Work out the finished part from the listing and answer in its coordinate system (mm). Face numbers are marked on the shaded views. A direction names the side the tool comes from. Give positions to 0.01 mm unless a question says otherwise; leave off trailing zeros. Write each loop counter-clockwise with the first axis right and the second up, starting at its lowest first coordinate (ties: lowest second). Pieces come first, ordered by that corner, then holes.
1) A tool of negligible diameter and unlimited length cuts with its end or side. For the marked faces 1, 2 and 3, from which of +Z, -Z, +X, -X, +Y, -Y can it reach the whole face along a straight path? Write none if from no direction.
2) Given pin 1 Ø8 at (y, z) = (19, 56) entering from +X; pin 2 Ø6 at (x, z) = (20, 60) entering from -Y; pin 3 Ø2 at (x, z) = (37.5, 40) entering from -Y, each flat-ended and moving along its own axis, determine where each tip first touches the part or whether it passes through.
3) Find section C-C (z = 43.5). Determine the outline of the cut face in (x, y).
4) Find section D-D (y = 76). Determine the outline of the cut face in (x, z), plus the area to 3 significant figures.
5) Find section A-A (z = 25). Determine the outline of the cut face in (x, y).
6) Find section B-B (y = 8). Determine the outline of the cut face in (x, z).
7) Straight lines are drawn through the part: probe 1 along Z at (x, y) = (-5.5, 17); probe 2 along Z at (x, y) = (-4, 13); probe 3 along X at (y, z) = (67, 14.5). For each, find the intervals that lie inside material, in ascending order.
Autodesk Inventor part; units mm, degrees
ref_plane "Work Plane1" through (0, 0, 62.5) normal (0, 0, -1) x (-1, 0, 0)
ref_plane "Work Plane2" through (-10, 0, 62.5) normal (-0.9866, 0.1632, 0) x (-0.1632, -0.9866, 0)
ref_plane "YZ Plane" through (0, 0, 0) normal (1, 0, 0) x (0, 1, 0)
sketch "Sketch1" plane through (0, 0, 0) normal (0, 0, 1) x (1, 0, 0)
  arc A0 (45, 98) -> (0, 0) centre (139.9137, -4.9145) ccw
  line L0 (45, 98) -> (45, 93)
  line L1 (0, 0) -> (5, 0)
  arc A1 (45, 93) -> (5, 0) centre (144.908, -5.0734) ccw
  dimension "d0" = 140
  dimension "d1" = 98
  dimension "d3" = 45
  dimension "d4" = 5
  dimension "d5" = 5
  dimension "d6" = 140
extrude "Extrusion1" add sketch "Sketch1" along normal blind 125
ref_plane "Work Plane1" through (0, 0, 62.5) normal (0, 0, -1) x (-1, 0, 0)
sketch "Sketch3" plane through (0, 0, 62.5) normal (0, 0, -1) x (-1, 0, 0)
  arc A0 (0, 0) -> (-45, 98) centre (-139.9137, -4.9145) ccw
  line L0 (0, 0) -> (10, 0)
  arc A1 (10, 0) -> (-45, 98) centre (-152.788, -26.9269) ccw
  arc A2 (0, 0) -> (-45, 98) centre (-139.9137, -4.9145) ccw
  dimension "d19" = 10
  dimension "d20" = 165
extrude "Extrusion3" add sketch "Sketch3" along normal mid plane 85
ref_plane "Work Plane2" through (-10, 0, 62.5) normal (-0.9866, 0.1632, 0) x (-0.1632, -0.9866, 0)
sketch "Sketch2" plane through (-10, 0, 62.5) normal (-0.9866, 0.1632, 0) x (-0.1632, -0.9866, 0)
  circle A0 centre (-20.6619, -35) radius 4
  circle A1 centre (-72.6619, -35) radius 4
  circle A2 centre (-20.6619, 35) radius 4
  circle A3 centre (-72.6619, 35) radius 4
  line L0 (0, 42.5) -> (0, -42.5)
  line L1 (-72.6619, 35) -> (-20.6619, 35) construction
  line L2 (-20.6619, 35) -> (-20.6619, -35) construction
  line L3 (-20.6619, -35) -> (-72.6619, -35) construction
  line L4 (-72.6619, -35) -> (-72.6619, 35) construction
  line L5 (-105.6619, -42.5) -> (-105.6619, 42.5)
  point P0 (0, 0)
  point P1 (-20.6619, 0)
  point P2 (0, 0)
  dimension "d9" = 8
  dimension "d10" = 8
  dimension "d12" = 52
  dimension "d14" = 8
  dimension "d15" = 8
  dimension "d16" = 70
  dimension "d23" = 33
extrude "Extrusion2" cut sketch "Sketch2" against normal through all
sketch "Sketch4" plane through (-10, 0, 62.5) normal (-0.9866, 0.1632, 0) x (-0.1632, -0.9866, 0)
  circle A0 centre (-38, 0) radius 5
  line L0 (0, 42.5) -> (0, -42.5)
  point P0 (-1.6319, -62.5)
  point P1 (0, 0)
  dimension "d24" = 10
  dimension "d25" = 38
extrude "Extrusion4" cut sketch "Sketch4" against normal through all
properties part number "SJ009" material "ABS Plastic"
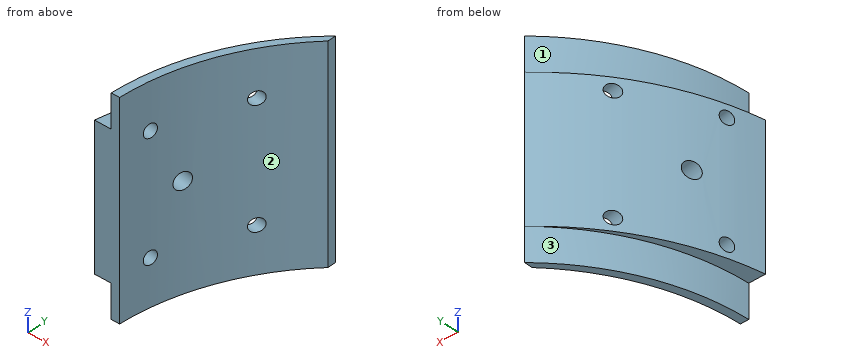
Results:
1. face 1: +Z, -X, +Y
1. face 2: +Z, -Z, +X, -Y
1. face 3: -Z, -X, +Y
2. pin 1: stops at x = 7.75
2. pin 2: stops at y = 51.84
2. pin 3: stops at y = 83.51
3. outline: (-10, 0) - (5, 0) arc R140 cw to (45, 93) - (45, 98) arc R165 ccw to start
4. outline: (23.83, 20) - (25.66, 20) - (25.66, 0) - (30.77, 0) - (30.77, 125) - (25.66, 125) - (25.66, 105) - (23.83, 105) - close
4. area: 795 mm2
5. outline: (-10, 0) - (5, 0) arc R140 cw to (6.36, 15.07) - (-6.22, 17.15) arc R165 ccw to start; (-4.42, 23.18) - (7.4, 21.23) arc R140 cw to (23.66, 64.92) - (16.51, 66.1) arc R165 ccw to start; (20.55, 71.76) - (27.16, 70.67) arc R140 cw to (45, 93) - (45, 98) arc R165 ccw to start
6. outline: (-8.47, 20) - (0.51, 20) - (0.51, 0) - (5.52, 0) - (5.52, 125) - (0.51, 125) - (0.51, 105) - (-8.47, 105) - close
7. probe 1: z = 20 to 25.04, 29.96 to 95.04, 99.96 to 105
7. probe 2: z = 20 to 105
7. probe 3: x = 19.8 to 24.89
